from build123d import *

# Parameters (mm, degrees)
F1_DEPTH = 1
F2_DEPTH = 8
F4_R     = 3.99999
F5_DEPTH = 5


# Not quite as in the source:
# - a fillet or chamfer is up to 0.001 mm smaller than in the source, because OpenCascade refuses the exact size


with BuildPart() as f1:
    # F0 (on Top) → F1 (new body)
    with BuildSketch(Plane.XY):
        with BuildLine():
            ThreePointArc((-24.6977130771, 2.8230095394), (-35.6977130771, 13.8230095394), (-46.6977130771, 2.8230095394))
            ThreePointArc((-46.6977130771, 2.8230095394), (-35.6977130771, -8.1769904606), (-24.6977130771, 2.8230095394))
        make_face()
        with BuildLine():
            ThreePointArc((-45.6977130771, 2.8230095394), (-35.6977130771, 12.8230095394), (-25.6977130771, 2.8230095394))
            ThreePointArc((-25.6977130771, 2.8230095394), (-35.6977130771, -7.1769904606), (-45.6977130771, 2.8230095394))
        make_face(mode=Mode.SUBTRACT)
    extrude(amount=F1_DEPTH)

    # F0 (on Top) → F2 (join)
    with BuildSketch(Plane.XY):
        with BuildLine():
            ThreePointArc((-58.6768434486, 3.3230095394), (-58.5012596634, 4.3457856294), (-58.1520691344, 5.3230095394))
            Line((-58.1520691344, 5.3230095394), (-66.6663400437, 5.3230095394))
            Line((-66.6663400437, 5.3230095394), (-66.6663400437, 3.3230095394))
            Line((-66.6663400437, 3.3230095394), (-61.1977130771, 3.3230095394))
            Line((-61.1977130771, 3.3230095394), (-58.6768434486, 3.3230095394))
        make_face()
        with BuildLine():
            Line((-66.6663400437, 0.3230095394), (-58.1520691344, 0.3230095394))
            ThreePointArc((-58.1520691344, 0.3230095394), (-58.5012596634, 1.3002334494), (-58.6768434486, 2.3230095394))
            Line((-58.6768434486, 2.3230095394), (-61.1977130771, 2.3230095394))
            Line((-61.1977130771, 2.3230095394), (-66.6663400437, 2.3230095394))
            Line((-66.6663400437, 2.3230095394), (-66.6663400437, 0.3230095394))
        make_face()
        with BuildLine():
            Line((-58.6768434486, 3.3230095394), (-56.6663400437, 3.3230095394))
            Line((-56.6663400437, 3.3230095394), (-56.6663400437, 5.3230095394))
            Line((-56.6663400437, 5.3230095394), (-58.1520691344, 5.3230095394))
            ThreePointArc((-58.1520691344, 5.3230095394), (-58.5012596634, 4.3457856294), (-58.6768434486, 3.3230095394))
        make_face()
        with BuildLine():
            Line((-56.6663400437, 0.3230095394), (-56.6663400437, 2.3230095394))
            Line((-56.6663400437, 2.3230095394), (-58.6768434486, 2.3230095394))
            ThreePointArc((-58.6768434486, 2.3230095394), (-58.5012596634, 1.3002334494), (-58.1520691344, 0.3230095394))
            Line((-58.1520691344, 0.3230095394), (-56.6663400437, 0.3230095394))
        make_face()
        with BuildLine():
            ThreePointArc((-56.6663400437, 3.3230095394), (-52.4472214269, 6.8151585763), (-48.6977130771, 2.8230095394))
            ThreePointArc((-48.6977130771, 2.8230095394), (-48.5498129284, 4.7783942616), (-48.109477783, 6.6892864159))
            ThreePointArc((-48.109477783, 6.6892864159), (-53.5065513921, 8.768241291), (-58.1520691344, 5.3230095394))
            Line((-58.1520691344, 5.3230095394), (-56.6663400437, 5.3230095394))
            Line((-56.6663400437, 5.3230095394), (-56.6663400437, 3.3230095394))
        make_face()
        with BuildLine():
            ThreePointArc((-48.109477783, -1.0432673371), (-48.5498129284, 0.8676248172), (-48.6977130771, 2.8230095394))
            ThreePointArc((-48.6977130771, 2.8230095394), (-52.4472214269, -1.1691394976), (-56.6663400437, 2.3230095394))
            Line((-56.6663400437, 2.3230095394), (-56.6663400437, 0.3230095394))
            Line((-56.6663400437, 0.3230095394), (-58.1520691344, 0.3230095394))
            ThreePointArc((-58.1520691344, 0.3230095394), (-53.5065513921, -3.1222222122), (-48.109477783, -1.0432673371))
        make_face()
        with BuildLine():
            ThreePointArc((-48.109477783, 6.6892864159), (-47.0616944573, 4.8809925611), (-46.6977130771, 2.8230095394))
            ThreePointArc((-46.6977130771, 2.8230095394), (-47.0616944573, 0.7650265177), (-48.109477783, -1.0432673371))
            ThreePointArc((-48.109477783, -1.0432673371), (-33.7423283549, -10.0290903119), (-22.6977130771, 2.8230095394))
            ThreePointArc((-22.6977130771, 2.8230095394), (-33.7423283549, 15.6751093907), (-48.109477783, 6.6892864159))
        make_face()
        with BuildLine():
            ThreePointArc((-24.6977130771, 2.8230095394), (-35.6977130771, -8.1769904606), (-46.6977130771, 2.8230095394))
            ThreePointArc((-46.6977130771, 2.8230095394), (-35.6977130771, 13.8230095394), (-24.6977130771, 2.8230095394))
        make_face(mode=Mode.SUBTRACT)
        with BuildLine():
            ThreePointArc((-48.109477783, -1.0432673371), (-47.0616944573, 0.7650265177), (-46.6977130771, 2.8230095394))
            Line((-46.6977130771, 2.8230095394), (-48.6977130771, 2.8230095394))
            ThreePointArc((-48.6977130771, 2.8230095394), (-48.5498129284, 0.8676248172), (-48.109477783, -1.0432673371))
        make_face()
        with BuildLine():
            Line((-48.6977130771, 2.8230095394), (-46.6977130771, 2.8230095394))
            ThreePointArc((-46.6977130771, 2.8230095394), (-47.0616944573, 4.8809925611), (-48.109477783, 6.6892864159))
            ThreePointArc((-48.109477783, 6.6892864159), (-48.5498129284, 4.7783942616), (-48.6977130771, 2.8230095394))
        make_face()
    extrude(amount=F2_DEPTH)

    # F4 (radius 4 in the source; OpenCascade refuses exactly that, so slightly less here)
    f4_edges = [f1.edges().sort_by_distance(p)[0] for p in [
        (-66.66634, 4.32301, 8),
        (-66.66634, 1.32301, 8),
        (-66.66634, 4.32301, 0),
        (-66.66634, 1.32301, 0),
    ]]
    fillet(f4_edges, radius=F4_R)

    # F3 (on face) → F5 (cut)
    with BuildSketch(Plane.XZ.offset(-0.3230095394)):
        with BuildLine():
            Line((-64.1663400437, 4), (-61.1663400437, 4))
            ThreePointArc((-61.1663400437, 4), (-62.6663400437, 5.5), (-64.1663400437, 4))
        make_face()
        with BuildLine():
            ThreePointArc((-64.1663400437, 4), (-62.6663400437, 2.5), (-61.1663400437, 4))
            Line((-61.1663400437, 4), (-64.1663400437, 4))
        make_face()
    extrude(amount=-F5_DEPTH, mode=Mode.SUBTRACT)


solid = f1.part
Check sheet for the modelled part. Datum: model origin and axes. Units: mm. A direction names the side the tool comes from. Round coordinates to 2 decimals unless told otherwise and drop trailing zeros. Order: outer loops, then holes, each group sorted by start corner. A loop starts at its lowest first (then second) coordinate and runs counter-clockwise, first axis right, second up.
(1) Scan lines: probe 1 along Y at (x, z) = (-59.5, 2.25); probe 2 along X at (y, z) = (6, 1.25); probe 3 along X at (y, z) = (1.5, 3.5). Record each from-to range of solid material in increasing order.
(2) Draft check along X on faces 1 (the flat face through (-33, -7, 1)), 2 (the flat face through (-60, 2.323, 4)), 3 (the cylindrical face through (-65.46, 1.31, 1.14)). Enter one of: pulls with the +X half, pulls with the -X half, needs draft (parallel to the pull), parting line crosses it, or undercut.
(3) Cross-section at A-A, the plane y = 10.5. Enter the section's corners in (x, z), and give its area (3 significant figures).
(4) Go/stop test with flat-tipped pins: P1, Ø4, axis at y = -4, z = 2, coming from the -X side; P2, Ø2.5, axis at x = -60.5, z = 2.5, coming from the +Y side; P3, Ø4, axis at x = -61.5, z = 5.5, coming from the -Y side. Record where each tip stops, or that it passes through.
(5) Cross-section at B-B, the plane z = 4.5. Enter the section's corners in (x, y).
(6) Access from +Z, -Z, +X, -X, +Y, -Y to the whole of each face (thin tool, end or side, straight path). Record for faces 4 (the flat face through (-61, 5.323, 5)), 5 (the cylindrical face through (-46.2, 6.1, 4.5)), 6 (the flat face through (-61, 3.323, 4)).
(7) Cross-section at C-C, the plane y = 7.5. Enter the section's corners in (x, z), and give its area (3 significant figures).
(8) Cross-section at D-D, the plane y = -5.5. Enter the section's corners in (x, z), and give its area (3 significant figures).
Check sheet entries:
1. probe 1: y = 0.32 to 2.32, 3.32 to 5.32
1. probe 2: x = -57.79 to -55.13, -50.27 to -46.23, -25.17 to -23.09
1. probe 3: x = -66.63 to -64.08, -61.25 to -56.47, -48.92 to -46.62, -24.78 to -22.77
2. face 1: undercut
2. face 2: needs draft
2. face 3: pulls with the -X half
3. outline: (-46.19, 0) - (-42.11, 0) - (-42.11, 1) - (-43.58, 1) - (-43.58, 8) - (-46.19, 8) - close; (-29.29, 0) - (-25.21, 0) - (-25.21, 8) - (-27.82, 8) - (-27.82, 1) - (-29.29, 1) - close
3. area: 44.7 mm2
4. P1: stops at x = -56.27
4. P2: stops at y = 5.32
4. P3: stops at y = 0.32
5. outline: (-66.63, 0.32) - (-64.08, 0.32) - (-64.08, 2.32) - (-66.63, 2.32) - close; (-66.63, 3.32) - (-64.08, 3.32) - (-64.08, 5.32) - (-66.63, 5.32) - close; (-61.25, 0.32) - (-58.15, 0.32) arc R6 ccw to (-48.11, -1.04) arc R13 ccw (long way) to (-48.11, 6.69) arc R6 ccw to (-58.15, 5.32) - (-61.25, 5.32) - (-61.25, 3.32) - (-56.67, 3.32) arc R4 cw (long way) to (-56.67, 2.32) - (-61.25, 2.32) - close; hole circle Ø22 at (-35.7, 2.82)
6. face 4: +Z, -Z, -X, +Y
6. face 5: +Z
6. face 6: +Z, -Z, -X
7. outline: (-56.46, 0) - (-48.94, 0) - (-48.94, 8) - (-56.46, 8) - close; (-47.83, 0) - (-44.54, 0) - (-44.54, 1) - (-45.65, 1) - (-45.65, 8) - (-47.83, 8) - close; (-26.86, 0) - (-23.57, 0) - (-23.57, 8) - (-25.74, 8) - (-25.74, 1) - (-26.86, 1) - close
7. area: 97.1 mm2
8. outline: (-45.68, 0) - (-41.24, 0) - (-41.24, 1) - (-42.89, 1) - (-42.89, 8) - (-45.68, 8) - close; (-30.15, 0) - (-25.71, 0) - (-25.71, 8) - (-28.51, 8) - (-28.51, 1) - (-30.15, 1) - close
8. area: 48.0 mm2
